Model file for the job. Use its own axes, mm. Face numbers are marked on the shaded views. A direction names the side the tool comes from. Give positions to 0.01 mm unless a question says otherwise; leave off trailing zeros. Write each loop counter-clockwise with the first axis right and the second up, starting at its lowest first coordinate (ties: lowest second). Pieces come first, ordered by that corner, then holes.
```python
from build123d import *

# Parameters (mm, degrees)
F0_R      = 63.5
F1_DEPTH  = 12.7
F2_R      = 38.1
F3_DEPTH  = 57.15
F4_R      = 50.8
F5_DEPTH  = 12.7
F6_R      = 6.35
F7_DEPTH  = 25.4
F8_R      = 6.35
F9_DEPTH  = 25.4
F10_R     = 6.35
F11_DEPTH = 25.4
F12_R     = 6.35
F13_DEPTH = 25.4
F14_W     = 50.8
F14_H     = 50.8
F15_DEPTH = 101.6


with BuildPart() as f1:
    # F0 (on Top) → F1 (new body)
    with BuildSketch(Plane.XY):
        with Locations((1.4321604976, 0)):
            Circle(F0_R)
    extrude(amount=F1_DEPTH)

    # F2 (on face) → F3 (join)
    with BuildSketch(Plane.XY.offset(12.7)):
        Circle(F2_R)
    extrude(amount=F3_DEPTH)

    # F4 (on face) → F5 (join)
    with BuildSketch(Plane.XY.offset(69.85)):
        Circle(F4_R)
    extrude(amount=F5_DEPTH)

    # F6 (on face) → F7 (cut)
    with BuildSketch(Plane(origin=(0, 0, 0), x_dir=(1, 0, 0), z_dir=(0, 0, -1))):
        with Locations((0, -55.4723255336)):
            Circle(F6_R)
    extrude(amount=-F7_DEPTH, mode=Mode.SUBTRACT)

    # F8 (on face) → F9 (cut)
    with BuildSketch(Plane.XY.offset(12.7)):
        with Locations((56.9999702275, 0)):
            Circle(F8_R)
    extrude(amount=-F9_DEPTH, mode=Mode.SUBTRACT)

    # F10 (on face) → F11 (cut)
    with BuildSketch(Plane(origin=(0, 0, 0), x_dir=(1, 0, 0), z_dir=(0, 0, -1))):
        with Locations((0, 56.2361478806)):
            Circle(F10_R)
    extrude(amount=-F11_DEPTH, mode=Mode.SUBTRACT)

    # F12 (on face) → F13 (cut)
    with BuildSketch(Plane(origin=(0, 0, 0), x_dir=(1, 0, 0), z_dir=(0, 0, -1))):
        with Locations((-55.0904199481, 0)):
            Circle(F12_R)
    extrude(amount=-F13_DEPTH, mode=Mode.SUBTRACT)

    # F14 (on face) → F15 (cut)
    with BuildSketch(Plane.XY.offset(82.55)):
        with Locations((1.4321604976, 0)):
            Rectangle(F14_W, F14_H)
    extrude(amount=-F15_DEPTH, mode=Mode.SUBTRACT)


solid = f1.part
```
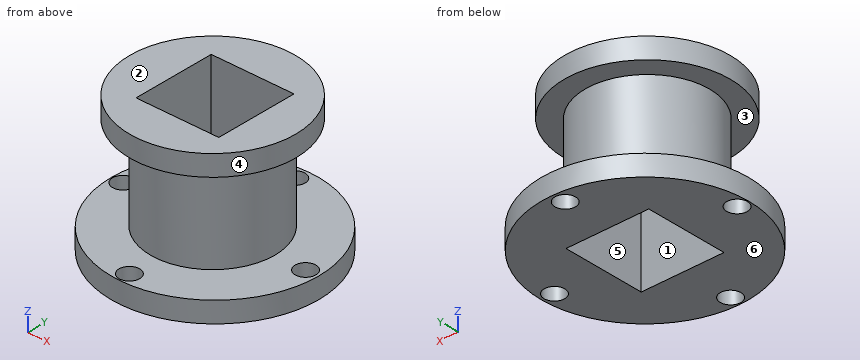
1. Pin check, flat tips, straight feed: P1, Ø7.5, axis at x = 57, y = 0, coming from the -Z side; P2, Ø11.5, axis at x = 0, y = -56.24, coming from the -Z side; P3, Ø15, axis at y = -2, z = 45, coming from the -X side; P4, Ø2, axis at x = 24, z = 55, coming from the +Y side. Stop position of each tip, or through.
Calculated:
P1: passes through
P2: stops at z = 69.85
P3: stops at x = -38.1
P4: stops at y = 30.37
2. Which spindle directions (+Z, -Z, +X, -X, +Y, -Y) get a long thin tool onto all of the face, cutting with end or side? Do the marked faces 1, 2 and 3. Say none if no direction does.
Calculated:
face 1: +Z, -Z
face 2: +Z, +X, -X, +Y, -Y
face 3: none
3. Pull direction X, two halves, no side cores. Call the marked faces 4, 5 and 6: +X half, -X half, draft (parallel to the pull), parting line (faces both ways), or undercut.
Calculated:
face 4: parting line
face 5: undercut
face 6: draft
4. Probe probe 1 along Y at (x, z) = (0, 3); probe 2 along X at (y, z) = (0.5, 10.5); probe 3 along X at (y, z) = (-5, 9) (3 decimals). List the from-to ranges inside material, lowest first.
Calculated:
probe 1: y = -63.48 to -62.59, -49.89 to -25.4, 25.4 to 49.12, 61.82 to 63.48
probe 2: x = -62.07 to -61.42, -48.76 to -23.97, 26.83 to 50.67, 63.33 to 64.93
probe 3: x = -61.871 to -59.005, -51.176 to -23.968, 26.832 to 53.086, 60.914 to 64.735
5. Slice it at C-C, the plane z = 42.5. Write the cut outline in (x, y), and give its area (3 significant figures).
Calculated:
outline: circle Ø76.2 at (0, 0); hole (-23.97, -25.4) - (26.83, -25.4) - (26.83, 25.4) - (-23.97, 25.4) - close
area: 1,980 mm2
6. Slice it at D-D, the plane x = 29. Write the cut outline in (y, z).
Calculated:
outline: (-57.2, 0) - (57.2, 0) - (57.2, 12.7) - (24.71, 12.7) - (24.71, 69.85) - (41.71, 69.85) - (41.71, 82.55) - (-41.71, 82.55) - (-41.71, 69.85) - (-24.71, 69.85) - (-24.71, 12.7) - (-57.2, 12.7) - close
7. Slice it at A-A, the plane y = 0. Write the cut outline in (x, z), and give its area (3 significant figures).
Calculated:
outline: (-62.07, 0) - (-61.44, 0) - (-61.44, 12.7) - (-62.07, 12.7) - close; (-50.8, 69.85) - (-38.1, 69.85) - (-38.1, 12.7) - (-48.74, 12.7) - (-48.74, 0) - (-23.97, 0) - (-23.97, 82.55) - (-50.8, 82.55) - close; (26.83, 0) - (50.65, 0) - (50.65, 12.7) - (38.1, 12.7) - (38.1, 69.85) - (50.8, 69.85) - (50.8, 82.55) - (26.83, 82.55) - close; (63.35, 0) - (64.93, 0) - (64.93, 12.7) - (63.35, 12.7) - close
area: 2,740 mm2
8. Slice it at B-B, the plane y = 18. Write the cut outline in (x, z).
Calculated:
outline: (-59.46, 0) - (-23.97, 0) - (-23.97, 82.55) - (-47.5, 82.55) - (-47.5, 69.85) - (-33.58, 69.85) - (-33.58, 12.7) - (-59.46, 12.7) - close; (26.83, 0) - (62.33, 0) - (62.33, 12.7) - (33.58, 12.7) - (33.58, 69.85) - (47.5, 69.85) - (47.5, 82.55) - (26.83, 82.55) - close
